Work out the finished part from the listing and answer in its coordinate system (mm). A direction names the side the tool comes from. Coordinates: 2 decimals unless noted, no trailing zeros. Write each loop counter-clockwise with the first axis right and the second up, starting at its lowest first coordinate (ties: lowest second). Pieces come first, ordered by that corner, then holes. Notation, with made-up numbers: M 25,-29 L 39,-29 A18 cw 39,-25 Z; hole C 5,20 d7. An arc over 180 degrees is marked long. Answer as CSV lines item,"result". Start each with the question number.
(1) Find the intervals of material crossed by L1, parallel to X at y = 4.25, z = 9 (3 decimals); L2, parallel to Y at x = 1.25, z = -4.75; L3, parallel to Z at x = 5.75, y = 11 (3 decimals), in increasing order. Write a range as [from, to].
(2) For faces 5 (the flat face through (-12, 4.05, 9)), 6 (the flat face through (3.445, 8, 8)), 7 (the flat face through (0, 3, 4.715)), 8 (the flat face through (-10, 1, -3)), determine the directions among +Z, -Z, +X, -X, +Y, -Y from which every point of the face is accessible in a straight line to the end or side of a thin tool.
(3) A cutting plane is placed at D-D on x = -4. Give the vertices of the cut face in (y, z) (3 decimals), then the cut area to 3 significant figures.
(4) A cutting plane is placed at A-A on y = 10.25. Give the vertices of the cut face in (x, z) (3 decimals), then the cut area to 3 significant figures.
(5) The mould has two halves that part along X. Classify faces 1 (the flat face through (0, 1, -11.115)), 2 (the flat face through (-3.445, 8, 8)), 3 (the cylindrical face through (-13.2, 2, 8)), 4 (the cylindrical face through (-9.399, 2.053, 9.823)): released by +X, released by -X, zero draft, split by the parting line, or undercut.
(6) A cutting plane is placed at C-C on z = -7.5. Give the vertices of the cut face in (x, y), then the cut area to 3 significant figures.
(7) A cutting plane is placed at B-B on x = 1.75. Give the vertices of the cut face in (y, z) (3 decimals).
(8) Flat-ended cylindrical pins translate along their axes: P1, Ø4, axis at x = -0.5, y = 6.5, coming from the +Z side; P2, Ø1.9, axis at y = 9, z = 6.5, coming from the +X side (3 decimals); P3, Ø5, axis at x = -1, y = 7.5, coming from the -Z side (3 decimals); P4, Ø8, axis at x = 1.5, z = -3.5, coming from the +Y side. Find the tip coordinate at first contact, or state that the pin passes through.
from build123d import *

# Parameters (mm, degrees)
BOSS_EXTRUDE1_DEPTH = 1.55
BOSS_EXTRUDE2_DEPTH = 2.5
SKETCH4_W           = 4.11
SKETCH4_H           = 6.4
BOSS_EXTRUDE3_DEPTH = 8
SKETCH6_R           = 2
CUT_EXTRUDE1_DEPTH  = 20.020600017


with BuildPart() as part:
    # Sketch1 → Boss-Extrude1 (new body)
    with BuildSketch(Plane(origin=(0, 0, 0), x_dir=(1, 0, 0), z_dir=(0, 1, 0))):
        with BuildLine():
            Line((10, -4.715), (10, 11.115))
            Line((10, 11.115), (-10, 11.115))
            Line((-10, 11.115), (-10, -4.715))
            ThreePointArc((-10, -4.715), (-13.2, -7.915), (-10, -11.115))
            Line((-10, -11.115), (10, -11.115))
            ThreePointArc((10, -11.115), (13.2, -7.915), (10, -4.715))
        make_face()
    extrude(amount=BOSS_EXTRUDE1_DEPTH)

    # Sketch3 → Boss-Extrude2 (add)
    with BuildSketch(Plane(origin=(0, 1.55, 0), x_dir=(1, 0, 0), z_dir=(0, 1, 0))):
        with BuildLine():
            Line((-10, -4.715), (10, -4.715))
            ThreePointArc((10, -4.715), (13.2, -7.915), (10, -11.115))
            Line((10, -11.115), (-10, -11.115))
            ThreePointArc((-10, -11.115), (-13.2, -7.915), (-10, -4.715))
        make_face()
    extrude(amount=BOSS_EXTRUDE2_DEPTH)

    # Sketch4 → Boss-Extrude3 (add)
    with BuildSketch(Plane(origin=(0, 4.05, 0), x_dir=(1, 0, 0), z_dir=(0, 1, 0))):
        with Locations((-5.5, -7.915)):
            Rectangle(SKETCH4_W, SKETCH4_H)
        with Locations((5.5, -7.915)):
            Rectangle(SKETCH4_W, SKETCH4_H)
    extrude(amount=BOSS_EXTRUDE3_DEPTH)

    # Sketch6 → Cut-Extrude1 (cut, through all)
    with BuildSketch(Plane(origin=(0, 4.05, 0), x_dir=(1, 0, 0), z_dir=(0, 1, 0))):
        with Locations(Location((-10, -7.915, 0), (0, 0, 270))):
            Circle(SKETCH6_R)
        with Locations(Location((10, -7.915, 0), (0, 0, 270))):
            Circle(SKETCH6_R)
    extrude(amount=-CUT_EXTRUDE1_DEPTH, mode=Mode.SUBTRACT)


solid = part.part
Here are the results:
1,L1,"x = [-7.555, -3.445], [3.445, 7.555]"
1,L2,"y = [0, 1.55]"
1,L3,"z = [4.715, 11.115]"
2,face 5,"+Z, -Z, -X, +Y"
2,face 6,"+Z, -Z, +Y"
2,face 7,"-Z, +X, -X, +Y"
2,face 8,"-Z, -X, +Y, -Y"
3,outline,"M 0,-11.115 L 1.55,-11.115 L 1.55,4.715 L 12.05,4.715 L 12.05,11.115 L 0,11.115 Z"
3,area,"102 mm^2"
4,outline,"M -7.555,4.715 L -3.445,4.715 L -3.445,11.115 L -7.555,11.115 Z; M 3.445,4.715 L 7.555,4.715 L 7.555,11.115 L 3.445,11.115 Z"
4,area,"52.6 mm^2"
5,face 1,"zero draft"
5,face 2,"undercut"
5,face 3,"released by -X"
5,face 4,"undercut"
6,outline,"M -10,0 L 10,0 L 10,1.55 L -10,1.55 Z"
6,area,"31.0 mm^2"
7,outline,"M 0,-11.115 L 1.55,-11.115 L 1.55,4.715 L 4.05,4.715 L 4.05,11.115 L 0,11.115 Z"
8,P1,"passes through"
8,P2,"stops at x = 7.555"
8,P3,"stops at z = 4.715"
8,P4,"stops at y = 1.55"
